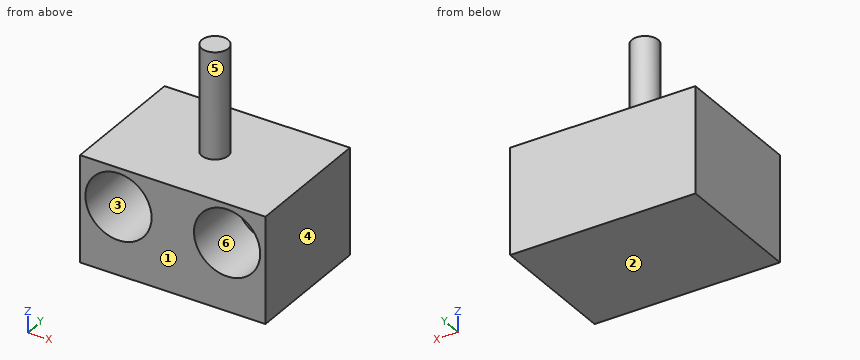
```python
from build123d import *

# Parameters (mm, degrees)
F0_W     = 70
F0_H     = 50
F1_DEPTH = 40
F2_R     = 5
F3_DEPTH = 40
F4_R     = 12.5
F5_DEPTH = 30
F6_R     = 12.5
F7_DEPTH = 25


with BuildPart() as f1:
    # F0 (on Top) → F1 (new body)
    with BuildSketch(Plane.XY):
        Rectangle(F0_W, F0_H)
    extrude(amount=F1_DEPTH)

    # F2 (on face) → F3 (join)
    with BuildSketch(Plane.XY.offset(40)):
        Circle(F2_R)
    extrude(amount=F3_DEPTH)

    # F4 (on face) → F5 (cut)
    with BuildSketch(Plane.XZ.offset(25)):
        with Locations((-20.5, 25.5)):
            Circle(F4_R)
    extrude(amount=-F5_DEPTH, mode=Mode.SUBTRACT)

    # F6 (on face) → F7 (cut)
    with BuildSketch(Plane.XZ.offset(25)):
        with Locations((20.5, 25.5)):
            Circle(F6_R)
    extrude(amount=-F7_DEPTH, mode=Mode.SUBTRACT)


solid = f1.part
```
Input: part model. Units: mm. Frame: model coordinates. Face numbers are marked on the shaded views. A direction names the side the tool comes from. Coordinates: 2 decimals unless noted, no trailing zeros. Write each loop counter-clockwise with the first axis right and the second up, starting at its lowest first coordinate (ties: lowest second). Pieces come first, ordered by that corner, then holes.
1) Material intervals for line 1 along X through (y, z) = (-15, 25); line 2 along Z through (x, y) = (-20.5, -17.75); line 3 along X through (y, z) = (-22, 32), sorted ascending.
2) Section D-D on y = 2. Output: boundary loops of the cut face in (x, z), and give its area (3 significant figures).
3) Set-up query: the marked faces 4, 5 and 6. Return all of +Z, -Z, +X, -X, +Y, -Y with unobstructed straight access to the full face (end or side cutting, diameter ignored); none if empty.
4) Section B-B on x = 0. Output: boundary loops of the cut face in (y, z), and give its area (3 significant figures).
5) Pin query (flat end, axial travel): pin 1 Ø6 at (x, y) = (1.5, 8.5) entering from +Z; pin 2 Ø3 at (x, z) = (5.5, 66) entering from -Y; pin 3 Ø12 at (x, z) = (-18.5, 19.5) entering from -Y; pin 4 Ø10 at (y, z) = (-11.5, 62.5) entering from -X. Return the tip coordinate at first contact, or that it passes through.
6) Section C-C on z = 22. Output: boundary loops of the cut face in (x, y).
7) Section A-A on y = -3. Output: boundary loops of the cut face in (x, z).
8) Mould query, pull axis Z, two halves, no side actions, for the marked faces 1, 2 and 3. Classes: pulls with the +Z half, pulls with the -Z half, needs draft (parallel to the pull), parting line crosses it, or undercut.
Check result:
1. line 1: x = -35 to -32.99, -8.01 to 8.01, 32.99 to 35
1. line 2: z = 0 to 13, 38 to 40
1. line 3: x = -35 to -31.18, -9.82 to 9.82, 31.18 to 35
2. outline: (-35, 0) - (35, 0) - (35, 40) - (4.58, 40) - (4.58, 80) - (-4.58, 80) - (-4.58, 40) - (-35, 40) - close; hole circle Ø25 at (-20.5, 25.5)
2. area: 2,680 mm2
3. face 4: +Z, -Z, +X, +Y, -Y
3. face 5: +Z
3. face 6: -Y
4. outline: (-25, 0) - (25, 0) - (25, 40) - (5, 40) - (5, 80) - (-5, 80) - (-5, 40) - (-25, 40) - close
4. area: 2,400 mm2
5. pin 1: stops at z = 40
5. pin 2: stops at y = -3
5. pin 3: stops at y = 5
5. pin 4: passes through
6. outline: (-35, -25) - (-32.5, -25) - (-32.5, 5) - (-8.5, 5) - (-8.5, -25) - (8.5, -25) - (8.5, 0) - (32.5, 0) - (32.5, -25) - (35, -25) - (35, 25) - (-35, 25) - close
7. outline: (-35, 0) - (35, 0) - (35, 40) - (4, 40) - (4, 80) - (-4, 80) - (-4, 40) - (-35, 40) - close; hole circle Ø25 at (-20.5, 25.5); hole circle Ø25 at (20.5, 25.5)
8. face 1: needs draft
8. face 2: pulls with the -Z half
8. face 3: undercut
